Could you check a few things on this model? Use its own coordinates, in mm. A direction names the side the tool comes from. Coordinates: 2 decimals unless noted, no trailing zeros. Write each loop counter-clockwise with the first axis right and the second up, starting at its lowest first coordinate (ties: lowest second). Pieces come first, ordered by that corner, then holes. Notation, with made-up numbers: (-2.75, -9.5) - (40.25, -9.5) arc R24 ccw to (40.25, 17.5) - close; hole circle Ø11 at (-14, 20.5). An arc over 180 degrees is marked (long way). Write item = value, one per line. Start each with the question number.
```python
from build123d import *

# Parameters (mm, degrees)
SKETCH1_R           = 6.35
SKETCH1_R_2         = 2.499995
BOSS_EXTRUDE1_DEPTH = 12.7
SKETCH2_W           = 1.567050356
SKETCH2_H           = 1.276855845
BOSS_EXTRUDE2_DEPTH = 2.54


with BuildPart() as part:
    # Sketch1 → Boss-Extrude1 (new body)
    with BuildSketch(Plane.XY):
        Circle(SKETCH1_R)
        Circle(SKETCH1_R_2, mode=Mode.SUBTRACT)
    extrude(amount=BOSS_EXTRUDE1_DEPTH)

    # Sketch2 → Boss-Extrude2 (add)
    with BuildSketch(Plane.XY.offset(12.7)):
        with Locations((0.164443556, 4.014357393)):
            Rectangle(SKETCH2_W, SKETCH2_H)
    extrude(amount=BOSS_EXTRUDE2_DEPTH)


solid = part.part
```
1) If I drill on probe 1 along Y at (x, z) = (0, 10.25); probe 2 along Z at (x, y) = (1.5, -3.75); probe 3 along X at (y, z) = (1.75, 9.5), over which ranges is the centre line in solid material (lowest first)? Write a range as [from, to].
2) Suppose I cut it at C-C on z = 10.5. Please give me the cut outline in (x, y), plus the area to 3 significant figures.
3) Which directions (+Z, -Z, +X, -X, +Y, -Y) give clear straight access to the entire face, cutting with the end or side of a thin tool? Please do faces 1 (the flat face through (0, 4.653, 14)), 2 (the flat face through (0.948, 4, 14)), 3 (the flat face through (-0.619, 4, 14)).
4) Suppose I cut it at A-A on y = 0. Please give me the cut outline in (x, z), plus the area to 3 significant figures.
5) Suppose I cut it at D-D on y = -2. Please give me the cut outline in (x, z), plus the area to 3 significant figures.
6) Suppose I cut it at B-B on x = 0. Please give me the cut outline in (y, z).
7) For P1, Ø1, axis at y = 3.5, z = 13.5, coming from the +X side; P2, Ø1, axis at x = -4, z = 11.5, coming from the -Y side; P3, Ø0.8, axis at x = 0, z = 14, coming from the -Y side, each with a flat end and sliding along its axis, tell me the tip position at first contact or that it passes through.
8) Thinking about a two-plate mould opening in Y: for faces 4 (the flat face through (0, 3.376, 14)), 5 (the flat face through (0, -3, 12.7)), 6 (the cylindrical face through (-0.33, 2.48, 6.26)), 7 (the cylindrical face through (-1.38, -6.2, 6.26)), which applies, +Y half, -Y half, draft (parallel to the pull), parting line (faces both ways), or undercut?
Reply:
q1.probe_1 = [-6.35, -2.5], [2.5, 6.35]
q1.probe_2 = [0, 12.7]
q1.probe_3 = [-6.1, -1.79], [1.79, 6.1]
q2.outline = circle Ø12.7 at (0, 0); hole circle Ø5 at (0, 0)
q2.area = 107 mm^2
q3.face_1 = +Z, +X, -X, +Y
q3.face_2 = +Z, +X, +Y, -Y
q3.face_3 = +Z, -X, +Y, -Y
q4.outline = (-6.35, 0) - (-2.5, 0) - (-2.5, 12.7) - (-6.35, 12.7) - close; (2.5, 0) - (6.35, 0) - (6.35, 12.7) - (2.5, 12.7) - close
q4.area = 97.8 mm^2
q5.outline = (-6.03, 0) - (-1.5, 0) - (-1.5, 12.7) - (-6.03, 12.7) - close; (1.5, 0) - (6.03, 0) - (6.03, 12.7) - (1.5, 12.7) - close
q5.area = 115 mm^2
q6.outline = (-6.35, 0) - (-2.5, 0) - (-2.5, 12.7) - (-6.35, 12.7) - close; (2.5, 0) - (6.35, 0) - (6.35, 12.7) - (4.65, 12.7) - (4.65, 15.24) - (3.38, 15.24) - (3.38, 12.7) - (2.5, 12.7) - close
q7.P1 = 0.95
q7.P2 = -5.3
q7.P3 = 3.38
q8.face_4 = -Y half
q8.face_5 = draft
q8.face_6 = undercut
q8.face_7 = parting line
